Model file for the job. Use its own axes, mm. A direction names the side the tool comes from. Coordinates: 2 decimals unless noted, no trailing zeros. Order: outer loops, then holes, each group sorted by start corner. A loop starts at its lowest first (then second) coordinate and runs counter-clockwise, first axis right, second up. Notation, with made-up numbers: M -31.5,-1 L 16.5,-1 A19 cw 16.5,26 Z; hole C 7,53.25 d7. An arc over 180 degrees is marked long. Return JSON: item names as keys, results as strings.
```python
from build123d import *

# Parameters (mm, degrees)
PROFILE_SKETCH_R      = 30
PROFILE_EXTRUDE_DEPTH = 15
HOLE_SKETCH_R         = 5.5
HOLE_CUT_DEPTH        = 70
GAP_CUT_DEPTH         = 10
GAP_CUT_DEPTH_BACK    = 10
GAP_SKETCH_W          = 15
GAP_SKETCH_H          = 15
UPPER_FILLET_RADIUS   = 7.5
UPPER_FILLET_LENGTH   = 25
LOWER_FILLET_RADIUS   = 7.5
LOWER_FILLET_LENGTH   = 25


with BuildPart() as part:
    # Profile Sketch → Profile Extrude (new body)
    with BuildSketch(Plane.XY):
        with BuildLine():
            Line((-60, 35), (0, 35))
            ThreePointArc((0, 35), (35, 0), (0, -35))
            Line((0, -35), (-60, -35))
            Line((-60, -35), (-60, 35))
        make_face()
        Circle(PROFILE_SKETCH_R, mode=Mode.SUBTRACT)
    extrude(amount=-PROFILE_EXTRUDE_DEPTH)

    # Hole Sketch → Hole Cut (cut)
    with BuildSketch(Plane(origin=(0, 35, 0), x_dir=(1, 0, 0), z_dir=(0, 1, 0))):
        with Locations(Location((-52.5, 7.5, 0), (0, 0, 180))):
            Circle(HOLE_SKETCH_R)
    extrude(amount=-HOLE_CUT_DEPTH, mode=Mode.SUBTRACT)

    # Gap Sketch → Gap Cut (cut, two sides: drawn at the far end of the back side and taken through both)
    with BuildSketch(Plane(origin=(0, 0, 0), x_dir=(1, 0, 0), z_dir=(0, 1, 0)).offset(-GAP_CUT_DEPTH_BACK)):
        with Locations((-52.5, 7.5)):
            Rectangle(GAP_SKETCH_W, GAP_SKETCH_H)
    extrude(amount=GAP_CUT_DEPTH + GAP_CUT_DEPTH_BACK, mode=Mode.SUBTRACT)

    # Upper Fillet: full round fillet: the end face becomes a half cylinder, R = half its width
    upper_fillet_face = Plane((-60, 22.5, -7.5), x_dir=(0, -1, 0), z_dir=(-1, 0, 0))  # on the end face: x along it, z out of the body
    upper_fillet_slab = upper_fillet_face.offset(-UPPER_FILLET_RADIUS / 2) * Box(UPPER_FILLET_LENGTH, 2 * UPPER_FILLET_RADIUS, UPPER_FILLET_RADIUS, mode=Mode.PRIVATE)  # the body's end, R deep
    upper_fillet_round = Plane((-52.5, 22.5, -7.5), x_dir=(-1, 0, 0), z_dir=(0, -1, 0)) * Cylinder(UPPER_FILLET_RADIUS, UPPER_FILLET_LENGTH, mode=Mode.PRIVATE)  # its axis R under the face
    add(upper_fillet_slab - upper_fillet_round, mode=Mode.SUBTRACT)

    # Lower Fillet: full round fillet: the end face becomes a half cylinder, R = half its width
    lower_fillet_face = Plane((-60, -22.5, -7.5), x_dir=(0, 1, 0), z_dir=(-1, 0, 0))  # on the end face: x along it, z out of the body
    lower_fillet_slab = lower_fillet_face.offset(-LOWER_FILLET_RADIUS / 2) * Box(LOWER_FILLET_LENGTH, 2 * LOWER_FILLET_RADIUS, LOWER_FILLET_RADIUS, mode=Mode.PRIVATE)  # the body's end, R deep
    lower_fillet_round = Plane((-52.5, -22.5, -7.5), x_dir=(-1, 0, 0), z_dir=(0, 1, 0)) * Cylinder(LOWER_FILLET_RADIUS, LOWER_FILLET_LENGTH, mode=Mode.PRIVATE)  # its axis R under the face
    add(lower_fillet_slab - lower_fillet_round, mode=Mode.SUBTRACT)


solid = part.part
```
Item 1: Pull direction Y, two halves, no side cores. Call faces 1 (the cylindrical face through (-29.97, 1.32, -7.4)), 2 (the cylindrical face through (-47.005, -22.325, -7.258)), 3 (the flat face through (-24, 35, -7)): +Y half, -Y half, draft (parallel to the pull), parting line (faces both ways), or undercut.
Check result:
{"face 1": "undercut", "face 2": "draft", "face 3": "+Y half"}
Item 2: 3-axis set-ups, long thin cutter, end or side, ignore diameter. For faces 4 (the flat face through (-48, 10, -4)), 5 (the flat face through (-28, 16, -15)): which of +Z, -Z, +X, -X, +Y, -Y reach the whole face in a straight line?
Check result:
{"face 4": "+Z, -Z, -X", "face 5": "-Z, +X, -X, +Y, -Y"}
Item 3: Saw through at D-D (x = -9.5). Write the cut outline in (y, z).
Check result:
{"outline": "M -35,-15 L -28.46,-15 L -28.46,0 L -35,0 Z; M 28.46,-15 L 35,-15 L 35,0 L 28.46,0 Z"}
Item 4: Wall check: line 1 (Y direction, x = -54, z = -13.5); line 2 (Z direction, x = -52.5, y = 16); line 3 (X direction, y = -14.5, z = -3.5). Give the ranges that are in metal, low to high.
Check result:
{"line 1": "y = -35 to -10, 10 to 35", "line 2": "z = -15 to -13, -2 to 0", "line 3": "x = -58.84 to -56.27, -48.73 to -26.26, 26.26 to 31.86"}
Item 5: Drop flat-ended pins along their axis: pin 1 Ø6.5 at (x, z) = (-52.5, -7.5) entering from +Y; pin 2 Ø5 at (y, z) = (-6.5, -4.5) entering from +X; pin 3 Ø4.5 at (y, z) = (-4, -4.5) entering from -X; pin 4 Ø1 at (y, z) = (-17.5, -12.5) entering from +X. Give the stop position or say it passes through.
Check result:
{"pin 1": "passes through", "pin 2": "stops at x = 34.77", "pin 3": "stops at x = -45", "pin 4": "stops at x = 30.59"}
Item 6: Saw through at C-C (x = -19). Write the cut outline in (y, z).
Check result:
{"outline": "M -35,-15 L -23.22,-15 L -23.22,0 L -35,0 Z; M 23.22,-15 L 35,-15 L 35,0 L 23.22,0 Z"}
Item 7: Saw through at A-A (z = -7.5). Write the cut outline in (x, y).
Check result:
{"outline": "M -60,-35 L -58,-35 L -58,-10 L -60,-10 Z; M -60,10 L -58,10 L -58,35 L -60,35 Z; M -47,-35 L 0,-35 A35 ccw 0,35 L -47,35 L -47,10 L -45,10 L -45,-10 L -47,-10 Z; hole C 0,0 d60"}
Item 8: Saw through at B-B (y = 11.5). Write the cut outline in (x, z).
Check result:
{"outline": "M -52.5,-15 L -27.71,-15 L -27.71,0 L -52.5,0 A7.5 ccw Z; M 27.71,-15 L 33.06,-15 L 33.06,0 L 27.71,0 Z; hole C -52.5,-7.5 d11"}
